Can you work these out from the model? Positions are in its coordinate system, mm. A direction names the side the tool comes from. Coordinates: 2 decimals unless noted, no trailing zeros. Order: outer loops, then holes, each group sorted by start corner. A loop starts at its lowest first (then second) coordinate and runs counter-clockwise, first axis right, second up. Notation, with made-up numbers: (-20.5, 59) -> (-9.5, 59) arc R28 cw to (-9.5, 80) -> close; hole circle Ø8 at (-9.75, 77). An arc over 180 degrees is marked (long way). Use a Markdown table: item, result. Add a question column.
1. Suppose I cut it at C-C, the plane z = 0.75. List the corners of the cut face in (x, y) for me (3 decimals).
2. We'd pull the mould along X, two halves only. Please class faces 1 (the flat face through (48, 14, 8)), 2 (the cylindrical face through (47.48, 29.16, 0.74)), 3 (the flat face through (0, 13, 3)): pulls with the +X half, pulls with the -X half, needs draft (parallel to the pull), parting line crosses it, or undercut.
3. If I drill on line 1 along Y through (x, z) = (4, 0.6) (3 decimals); line 2 along Z through (x, y) = (23.5, 9); line 3 along X through (y, z) = (30.5, 1.5), over which ranges is the centre line in solid material (lowest first)? Write a range as from..to.
4. Suppose I cut it at D-D, the plane x = 30.8. List the corners of the cut face in (y, z) for me (3 decimals).
5. For pin 1 Ø4 at (x, z) = (29, 7) entering from +Y; pin 2 Ø5 at (x, y) = (4, 29.625) entering from +Z; pin 3 Ø3 at (y, z) = (5.5, 4) entering from -X, each with a flat end and sliding along its axis, tell me the tip position at first contact or that it passes through.
6. Suppose I cut it at A-A, the plane x = 46. List the corners of the cut face in (y, z) for me (3 decimals), then the cut area to 3 significant figures.
7. For faces 4 (the flat face through (3, 15, 8)), 5 (the flat face through (50, 13, 3)), 6 (the flat face through (25, 18, 3.5)), 7 (the flat face through (25, 17, 8)), 8 (the flat face through (25, 8, 8.6)), which set-ups out of +Z, -Z, +X, -X, +Y, -Y let a thin tool reach every point of the face, with its end or its side?
8. Suppose I cut it at B-B, the plane y = 7. List the corners of the cut face in (x, z) for me.
Autodesk Inventor part; units mm, degrees
ref_plane "YZ Plane" through (0, 0, 0) normal (1, 0, 0) x (0, 1, 0)
ref_plane "XZ Plane" through (0, 0, 0) normal (0, 1, 0) x (-1, 0, 0)
ref_plane "XY Plane" through (0, 0, 0) normal (0, 0, 1) x (1, 0, 0)
sketch "Sketch1" plane through (0, 0, 0) normal (0, 0, 1) x (1, 0, 0)
  line L0 (0, 0) -> (50, 0)
  line L1 (50, 0) -> (50, 34)
  line L2 (50, 34) -> (0, 34)
  line L3 (0, 34) -> (0, 0)
  circle A0 centre (4, 29.625) radius 1.55
  circle A1 centre (19.2, 29.625) radius 1.55
  circle A2 centre (30.8, 29.625) radius 1.55
  circle A3 centre (46, 29.625) radius 1.55
  dimension "d0" = 50
  dimension "d1" = 34
  dimension "d2" = 4.375
  dimension "d3" = 4.375
  dimension "d4" = 4.375
  dimension "d5" = 4.375
  dimension "d6" = 15.2
  dimension "d7" = 15.2
  dimension "d8" = 34
  dimension "d9" = 4
  dimension "d10" = 4
  dimension "d11" = 3.1
  dimension "d12" = 3.1
  dimension "d13" = 3.1
  dimension "d14" = 3.1
extrude "Extrusion1" add sketch "Sketch1" along normal blind 3.5
sketch "Sketch2" plane through (0, 0, 3.5) normal (0, 0, 1) x (1, 0, 0)
  line L0 (0, 2) -> (50, 2)
  line L1 (50, 2) -> (50, 0)
  line L2 (50, 0) -> (0, 0)
  line L3 (0, 0) -> (0, 2)
  line L4 (0, 0) -> (50, 0)
  line L5 (0, 34) -> (0, 0)
  line L6 (50, 0) -> (50, 34)
  dimension "d17" = 2
extrude "Extrusion2" add sketch "Sketch2" along normal blind 5.1
sketch "Sketch3" plane through (0, 2, 3.5) normal (0, 1, 0) x (1, 0, 0)
  line L0 (0, -5.1) -> (50, -5.1)
  line L1 (50, -5.1) -> (50, -3.1)
  line L2 (50, -3.1) -> (0, -3.1)
  line L3 (0, -3.1) -> (0, -5.1)
  line L4 (0, 0) -> (0, -5.1)
  line L5 (50, 0) -> (50, -5.1)
  line L6 (50, -5.1) -> (0, -5.1)
  line L7 (50, 0) -> (0, 0)
  point P0 (0, 3.5)
  dimension "d20" = 3.1
extrude "Extrusion3" add sketch "Sketch3" along normal blind 15 contours L3 L2 L1 L0
chamfer "Chamfer1" distance 5 angle 45 2 edges at (50, 17, 7.6) (0, 17, 7.6)
chamfer "Chamfer2" distance 2 angle 45 4 edges at (2.45, 29.625, 3.5) (17.65, 29.625, 3.5) (29.25, 29.625, 3.5) (44.45, 29.625, 3.5)
chamfer "Chamfer3" distance 1 angle 45 2 edges at (0, 34, 1.75) (50, 34, 1.75)
properties part number "HX711MountingBracketv2"
Worked out:
| question | item | result |
|---|---|---|
| 1 | outline | (0, 0) -> (50, 0) -> (50, 33) -> (49, 34) -> (1, 34) -> (0, 33) -> close; hole circle Ø3.1 at (4, 29.625); hole circle Ø3.1 at (19.2, 29.625); hole circle Ø3.1 at (30.8, 29.625); hole circle Ø3.1 at (46, 29.625) |
| 2 | face 1 | pulls with the +X half |
| 2 | face 2 | undercut |
| 2 | face 3 | pulls with the -X half |
| 3 | line 1 | y = 0..28.075, 31.175..34 |
| 3 | line 2 | z = 0..3.5, 6.6..8.6 |
| 3 | line 3 | x = 0..2.72, 5.28..17.92, 20.48..29.52, 32.08..44.72, 47.28..50 |
| 4 | outline | (0, 0) -> (28.075, 0) -> (28.075, 1.5) -> (26.075, 3.5) -> (2, 3.5) -> (2, 6.6) -> (17, 6.6) -> (17, 8.6) -> (0, 8.6) -> close; (31.175, 0) -> (34, 0) -> (34, 3.5) -> (33.175, 3.5) -> (31.175, 1.5) -> close |
| 5 | pin 1 | stops at y = 17 |
| 5 | pin 2 | stops at z = 2.45 |
| 5 | pin 3 | stops at x = 0 |
| 6 | outline | (0, 0) -> (28.075, 0) -> (28.075, 1.5) -> (26.075, 3.5) -> (2, 3.5) -> (2, 6.6) -> (16, 6.6) -> (16, 8.6) -> (0, 8.6) -> close; (31.175, 0) -> (34, 0) -> (34, 3.5) -> (33.175, 3.5) -> (31.175, 1.5) -> close |
| 6 | area | 142 mm² |
| 7 | face 4 | +Z, -X, +Y |
| 7 | face 5 | +Z, -Z, +X, +Y, -Y |
| 7 | face 6 | +X, -X, +Y |
| 7 | face 7 | +Z, +X, -X, +Y |
| 7 | face 8 | +Z, +X, -X, +Y, -Y |
| 8 | outline | (0, 0) -> (50, 0) -> (50, 3.5) -> (0, 3.5) -> close; (0, 6.6) -> (50, 6.6) -> (50, 8.6) -> (0, 8.6) -> close |
